Work out the finished part from the listing and answer in its coordinate system (mm). A direction names the side the tool comes from. Round coordinates to 2 decimals unless told otherwise and drop trailing zeros. Loops run counter-clockwise (first coordinate to the right, second up) from the corner with the lowest first, then second, coordinate; pieces in that order, holes last. Notation, with made-up numbers: M 60.25,40.5 L 80.25,40.5 A20 ccw 80.25,65.5 Z; hole C 89.25,81.25 d3. An arc over 180 degrees is marked long. One line per item, written item: value.
```python
from build123d import *

# Parameters (mm, degrees)
SKETCH1_W           = 12
SKETCH1_H           = 12
BOSS_EXTRUDE1_DEPTH = 6
SKETCH3_W           = 12
SKETCH3_H           = 9.5
CUT_EXTRUDE1_DEPTH  = 1
SKETCH4_W           = 3
SKETCH4_H           = 9.5
BOSS_EXTRUDE2_DEPTH = 0.5
SKETCH6_R           = 3
BOSS_EXTRUDE3_DEPTH = 3.5
SKETCH7_R           = 1.85
CUT_EXTRUDE2_DEPTH  = 21.5
SKETCH8_W           = 1.2
SKETCH8_H           = 1
SKETCH8_W_2         = 1
SKETCH8_H_2         = 1.2
BOSS_EXTRUDE4_DEPTH = 4


with BuildPart() as part:
    # Sketch1 → Boss-Extrude1 (new body)
    with BuildSketch(Plane(origin=(0, 0, 0), x_dir=(1, 0, 0), z_dir=(0, 1, 0))):
        with Locations((-6, 6)):
            Rectangle(SKETCH1_W, SKETCH1_H)
    extrude(amount=BOSS_EXTRUDE1_DEPTH)

    # Sketch3 → Cut-Extrude1 (cut)
    with BuildSketch(Plane(origin=(0, 6, 0), x_dir=(1, 0, 0), z_dir=(0, 1, 0))):
        with Locations((-6, 4.75)):
            Rectangle(SKETCH3_W, SKETCH3_H)
    extrude(amount=-CUT_EXTRUDE1_DEPTH, mode=Mode.SUBTRACT)

    # Sketch4 → Boss-Extrude2 (add)
    with BuildSketch(Plane(origin=(0, 5, 0), x_dir=(1, 0, 0), z_dir=(0, 1, 0))):
        with Locations((-6, 4.75)):
            Rectangle(SKETCH4_W, SKETCH4_H)
    extrude(amount=BOSS_EXTRUDE2_DEPTH)

    # Sketch6 → Boss-Extrude3 (add)
    with BuildSketch(Plane(origin=(0, 0, -12), x_dir=(-1, 0, 0), z_dir=(0, 0, -1))):
        with Locations(Location((6, 3, 0), (0, 0, 270))):
            Circle(SKETCH6_R)
    extrude(amount=BOSS_EXTRUDE3_DEPTH)

    # Sketch7 → Cut-Extrude2 (cut, through all)
    with BuildSketch(Plane(origin=(0, 0, -15.5), x_dir=(-1, 0, 0), z_dir=(0, 0, -1))):
        with Locations((6, 3)):
            Circle(SKETCH7_R)
    extrude(amount=-CUT_EXTRUDE2_DEPTH, mode=Mode.SUBTRACT)

    # Sketch8 → Boss-Extrude4 (add)
    with BuildSketch(Plane.XZ):
        with Locations((-8.9, -11.5)):
            Rectangle(SKETCH8_W, SKETCH8_H)
        with Locations((-10.686701077, -0.6)):
            Rectangle(SKETCH8_W_2, SKETCH8_H_2)
        with Locations((-0.6, -0.5)):
            Rectangle(SKETCH8_W, SKETCH8_H)
        with Locations((-9, -2.967121794)):
            Rectangle(SKETCH8_W_2, SKETCH8_H_2)
    extrude(amount=BOSS_EXTRUDE4_DEPTH)


solid = part.part
```
1) Find section B-B (z = -6.5). Give the vertices of the cut face in (x, y).
Check values:
outline: M -12,0 L 0,0 L 0,5 L -4.5,5 L -4.5,5.5 L -7.5,5.5 L -7.5,5 L -12,5 Z; hole C -6,3 d3.7
2) Find section C-C (x = -2.5). Give the vertices of the cut face in (y, z), then the cut area to 3 significant figures.
Check values:
outline: M 0,-12 L 6,-12 L 6,-9.5 L 5,-9.5 L 5,0 L 0,0 Z
area: 62.5 mm2
3) Find section A-A (y = 3). Give the vertices of the cut face in (x, z), then the cut area to 3 significant figures.
Check values:
outline: M -12,-12 L -9,-12 L -9,-15.5 L -7.85,-15.5 L -7.85,0 L -12,0 Z; M -4.15,-15.5 L -3,-15.5 L -3,-12 L 0,-12 L 0,0 L -4.15,0 Z
area: 108 mm2
4) For faces 4 (the face through (-1, -2, -1)), 5 (the face through (-8.3, -2, -11.5)), 6 (the face through (-11.187, -2, -1)), determine the directions among +Z, -Z, +X, -X, +Y, -Y from which every point of the face is accessible in a straight line to the end or side of a thin tool.
Check values:
face 4: -Z, +X, -Y
face 5: +Z, -Z, +X, -Y
face 6: +Z, -Z, -X, -Y
5) The mould has two halves that part along Z. Classify faces 1 (the face through (-10, 2, -12)), 2 (the face through (-9, -2, -3.567)), 3 (the face through (-11, -4, -1)): +Z half, -Z half, draft (parallel to the pull), parting line (faces both ways), or undercut.
Check values:
face 1: -Z half
face 2: undercut
face 3: draft
6) Each of these flat-tipped pins is pushed along its axis until it touches: pin 1 (5 mm diameter, centred on x = -4.5, y = -1.5, fed in from +Z); pin 2 (0.5 mm diameter, centred on x = -9, y = -1.5, fed in from +Z); pin 3 (1.1 mm diameter, centred on y = -2, z = -0.5, fed in from -X); pin 4 (3.5 mm diameter, centred on x = -9.5, z = -3.5, fed in from +Y). Where does it stop, or does it pass through?
Check values:
pin 1: z = 0
pin 2: z = -2.37
pin 3: x = -11.19
pin 4: y = 5
7) Find section D-D (x = -5). Give the vertices of the cut face in (y, z).
Check values:
outline: M 0,-12 L 0.17,-12 L 0.17,-15.5 L 1.44,-15.5 L 1.44,0 L 0,0 Z; M 4.56,-15.5 L 5.83,-15.5 L 5.83,-12 L 6,-12 L 6,-9.5 L 5.5,-9.5 L 5.5,0 L 4.56,0 Z
8) Find the intervals of material crossed by probe 1 along Y at (x, z) = (-6, -4.25); probe 2 along Y at (x, z) = (-11, -5.25); probe 3 along Z at (x, y) = (-11, 3.25), in increasing order. Write a range as from..to.
Check values:
probe 1: 0..1.15, 4.85..5.5
probe 2: 0..5
probe 3: -12..0
